from build123d import *

# Parameters (mm, degrees)
SKETCH_W        = 30
SKETCH_H        = 20
PAD_DEPTH       = 2
SKETCH001_R     = 1.3
POCKET_DEPTH    = 5
POCKET001_DEPTH = 5


with BuildPart() as part:
    # Sketch → Pad (new body)
    with BuildSketch(Plane.XY):
        Rectangle(SKETCH_W, SKETCH_H)
    extrude(amount=PAD_DEPTH)

    # Sketch001 (on Face6 of Pad) → Pocket (cut)
    with BuildSketch(Plane.XY.offset(2)):
        with Locations((-10, 4.7)):
            Circle(SKETCH001_R)
        with Locations((-10, -4.7)):
            Circle(SKETCH001_R)
    extrude(amount=-POCKET_DEPTH, mode=Mode.SUBTRACT)

    # Sketch001 (on Face6 of Pad) → Pocket001 (cut)
    with BuildSketch(Plane.XY.offset(2)):
        with Locations((-10, 4.7)):
            Circle(SKETCH001_R)
        with Locations((-10, -4.7)):
            Circle(SKETCH001_R)
    extrude(amount=-POCKET001_DEPTH, mode=Mode.SUBTRACT)


solid = part.part
Read the model definition and answer for the solid it produces. Units are mm, in the model's axes. Give positions to 0.01 mm unless a question says otherwise; leave off trailing zeros. Write each loop counter-clockwise with the first axis right and the second up, starting at its lowest first coordinate (ties: lowest second). Pieces come first, ordered by that corner, then holes. Notation, with made-up numbers: M 60.5,54.25 L 111.5,54.25 A19 ccw 111.5,86.25 Z; hole C -24.75,81 d3. An arc over 180 degrees is marked long. One line per item, written item: value. Start each with the question number.
(1) Find section B-B (z = 0.35). Determine the outline of the cut face in (x, y), plus the area to 3 significant figures.
(2) Find section C-C (x = -10). Determine the outline of the cut face in (y, z).
(3) Determine the mould class of faces 1 (the flat face through (0, 0, 2)), 2 (the cylindrical face through (-8.76, -4.31, 1.01)), 3 (the flat face through (0, 10, 1)), 4 (the cylindrical face through (-8.8, 4.2, 1)) for opening direction Y: pulls with the +Y half, pulls with the -Y half, needs draft (parallel to the pull), parting line crosses it, or undercut.
(4) Find section A-A (y = 4.7). Determine the outline of the cut face in (x, z), plus the area to 3 significant figures.
(5) A flat-ended cylindrical pin translates along its axis: pin 1 Ø2.5 at (x, y) = (-10, 4.7) entering from +Z. Find the tip coordinate at first contact, or state that the pin passes through.
(6) Find section D-D (y = -5.25). Determine the outline of the cut face in (x, z).
(7) Find the intervals of material crossed by line 1 (Y direction, x = -10, z = 1.1); line 2 (X direction, y = 4.75, z = 0.95); line 3 (X direction, y = 4.25, z = 0.85), in increasing order.
Results below:
1. outline: M -15,-10 L 15,-10 L 15,10 L -15,10 Z; hole C -10,-4.7 d2.6; hole C -10,4.7 d2.6
1. area: 589 mm^2
2. outline: M -10,0 L -6,0 L -6,2 L -10,2 Z; M -3.4,0 L 3.4,0 L 3.4,2 L -3.4,2 Z; M 6,0 L 10,0 L 10,2 L 6,2 Z
3. face 1: needs draft
3. face 2: undercut
3. face 3: pulls with the +Y half
3. face 4: undercut
4. outline: M -15,0 L -11.3,0 L -11.3,2 L -15,2 Z; M -8.7,0 L 15,0 L 15,2 L -8.7,2 Z
4. area: 54.8 mm^2
5. pin 1: passes through
6. outline: M -15,0 L -11.18,0 L -11.18,2 L -15,2 Z; M -8.82,0 L 15,0 L 15,2 L -8.82,2 Z
7. line 1: y = -10 to -6, -3.4 to 3.4, 6 to 10
7. line 2: x = -15 to -11.3, -8.7 to 15
7. line 3: x = -15 to -11.22, -8.78 to 15
